```python
from build123d import *

# Parameters (mm, degrees)
SKETCH2_R           = 10
BOSS_EXTRUDE2_DEPTH = 10
SKETCH3_R           = 6.4
BOSS_EXTRUDE3_DEPTH = 7.9
SKETCH4_R           = 2.75
CUT_EXTRUDE1_DEPTH  = 5
FILLET1_R           = 2


with BuildPart() as part:
    # Sketch2 → Boss-Extrude2 (new body)
    with BuildSketch(Plane(origin=(0, 0, 0), x_dir=(1, 0, 0), z_dir=(0, 1, 0))):
        Circle(SKETCH2_R)
        with BuildLine():
            Line((-10, 75), (-10, 0))
            ThreePointArc((-10, 0), (0, 10), (10, 0))
            Line((10, 0), (10, 75))
            Line((10, 75), (-10, 75))
        make_face()
    extrude(amount=BOSS_EXTRUDE2_DEPTH)

    # Sketch3 → Boss-Extrude3 (add)
    with BuildSketch(Plane(origin=(0, 10, 0), x_dir=(1, 0, 0), z_dir=(0, 1, 0))):
        Circle(SKETCH3_R)
    extrude(amount=BOSS_EXTRUDE3_DEPTH)

    # Sketch4 → Cut-Extrude1 (cut)
    with BuildSketch(Plane(origin=(0, 0, -75), x_dir=(-1, 0, 0), z_dir=(0, 0, -1))):
        with Locations((0, 5)):
            Circle(SKETCH4_R)
    extrude(amount=-CUT_EXTRUDE1_DEPTH, mode=Mode.SUBTRACT)

    # Fillet1
    fillet1_edges = [part.edges().sort_by_distance(p)[0] for p in [
        (10, 10, -37.5),
        (0, 10, -75),
        (-10, 10, -37.5),
        (0, 10, 10),
        (-10, 0, -37.5),
        (0, 0, -75),
        (10, 0, -37.5),
        (0, 0, 10),
        (-10, 5, -75),
        (10, 5, -75),
    ]]
    fillet(fillet1_edges, radius=FILLET1_R)


solid = part.part
```
Work out the finished part from the listing and answer in its coordinate system (mm). A direction names the side the tool comes from. Coordinates: 2 decimals unless noted, no trailing zeros. Write each loop counter-clockwise with the first axis right and the second up, starting at its lowest first coordinate (ties: lowest second). Pieces come first, ordered by that corner, then holes.
Q1. A cutting plane is placed at C-C, the plane x = 0. Give the vertices of the cut face in (y, z).
Q2. Which of the six approach directions +Z, -Z, +X, -X, +Y, -Y give full straight-line access (tool end or side, diameter ignored) to faces 5 (the face through (-10, 5, -37)), 6 (the face through (-5.08, 13.89, 3.89))?
Q3. Find the intervals of material crossed by line 1 (Y direction, x = 0, z = -71.8); line 2 (Y direction, x = -2.5, z = -46); line 3 (X direction, y = 1, z = -14), in increasing order.
Q4. A cutting plane is placed at B-B, the plane z = -51. Give the vertices of the cut face in (x, y), then the cut area to 3 significant figures.
Q5. Each of these flat-tipped pins is pushed along its axis until it touches: pin 1 Ø3 at (x, y) = (6.5, 10.5) entering from -Z; pin 2 Ø8 at (x, z) = (2.5, -64) entering from +Y; pin 3 Ø2 at (y, z) = (9, 1) entering from -X. Where does it stop, or does it pass through?
Q6. A cutting plane is placed at A-A, the plane y = 5. Give the vertices of the cut face in (x, z), then the cut area to 3 significant figures.
Q7. Determine the mould class of faces 1 (the face through (0, 10, -42)), 2 (the face through (0, 5, -70)), 3 (the face through (10, 5, -36)), 4 (the face through (0.596, 2.315, -72.535)) for opening direction Y: released by +Y, released by -Y, zero draft, split by the parting line, or undercut.
Findings below:
1. outline: (0, -73) arc R2 ccw to (2, -75) - (2.25, -75) - (2.25, -70) - (7.75, -70) - (7.75, -75) - (8, -75) arc R2 ccw to (10, -73) - (10, -6.4) - (17.9, -6.4) - (17.9, 6.4) - (10, 6.4) - (10, 8) arc R2 ccw to (8, 10) - (2, 10) arc R2 ccw to (0, 8) - close
2. face 5: +Z, -Z, -X, +Y, -Y
2. face 6: +Y
3. line 1: y = 0 to 2.25, 7.75 to 10
3. line 2: y = 0 to 10
3. line 3: x = -9.73 to 9.73
4. outline: (-10, 2) arc R2 ccw to (-8, 0) - (8, 0) arc R2 ccw to (10, 2) - (10, 8) arc R2 ccw to (8, 10) - (-8, 10) arc R2 ccw to (-10, 8) - close
4. area: 197 mm2
5. pin 1: stops at z = -74.73
5. pin 2: stops at y = 10
5. pin 3: stops at x = -9.98
6. outline: (-10, -73) arc R2 ccw to (-8, -75) - (-2.75, -75) - (-2.75, -70) - (2.75, -70) - (2.75, -75) - (8, -75) arc R2 ccw to (10, -73) - (10, 0) arc R10 ccw to (-10, 0) - close
6. area: 1,630 mm2
7. face 1: released by +Y
7. face 2: undercut
7. face 3: zero draft
7. face 4: undercut
